Work out the finished part from the listing and answer in its coordinate system (mm). A direction names the side the tool comes from. Coordinates: 2 decimals unless noted, no trailing zeros. Loops run counter-clockwise (first coordinate to the right, second up) from the corner with the lowest first, then second, coordinate; pieces in that order, holes last. Notation, with made-up numbers: (-5.75, -33) - (43.25, -33) arc R14 ccw to (43.25, -6) - close; hole circle Ø2 at (42, -38). An arc over 180 degrees is marked (long way). Write each question's results on one line, items separated by ' | '. Start each with the question number.
Item 1: A tool of negligible diameter and unlimited length cuts with its end or side. For faces 1 (the face through (0, 1, -1)), 2 (the face through (0, 0, -3)), 3 (the face through (0, 1, 81)), from which of +Z, -Z, +X, -X, +Y, -Y can it reach the whole face along a straight path? Write none if from no direction.
Item 2: Each of these flat-tipped pins is pushed along its axis until it touches: pin 1 Ø1.5 at (x, z) = (-0.5, 46) entering from +Y; pin 2 Ø2 at (x, z) = (1.5, 39.5) entering from +Y. Where does it stop, or does it pass through?
Item 3: Section C-C, the plane z = 68.5 is taken. Write down the section's boundary in (x, y).
Item 4: Section A-A, the plane y = 0 is taken. Write down the section's boundary in (x, z), plus the area to 3 significant figures.
Item 5: Consider probe 1 along Z at (x, y) = (0.95, -1.05); probe 2 along X at (y, z) = (-0.15, 50). Determine where each line is inside the solid, lowest interval first. Write a range as [from, to].
Autodesk Inventor part; units mm, degrees
ref_plane "YZ Plane" through (0, 0, 0) normal (1, 0, 0) x (0, 1, 0)
ref_plane "XZ Plane" through (0, 0, 0) normal (0, 1, 0) x (-1, 0, 0)
ref_plane "XY Plane" through (0, 0, 0) normal (0, 0, 1) x (1, 0, 0)
sketch "Sketch1" plane through (0, 0, 0) normal (0, 0, 1) x (1, 0, 0)
  circle A0 centre (0, 0) radius 2.5
  dimension "d0" = 5
extrude "Extrusion1" add sketch "Sketch1" along normal blind 80
sketch "Sketch2" plane through (0, 0, 80) normal (0, 0, 1) x (1, 0, 0)
  circle A0 centre (0, 0) radius 2.5
  circle A1 centre (0, 0) radius 1
  dimension "d3" = 2
extrude "Extrusion2" add sketch "Sketch2" along normal blind 3 contours A1
sketch "Sketch3" plane through (0, 0, 0) normal (0, 0, -1) x (-1, 0, 0)
  circle A0 centre (0, 0) radius 1
  dimension "d6" = 2
extrude "Extrusion3" add sketch "Sketch3" along normal blind 3
properties part number "Bone-8cm"
Answer key:
1) face 1: -Z | face 2: -Z, +X, -X, +Y, -Y | face 3: +Z
2) pin 1: stops at y = 2.5 | pin 2: stops at y = 2.45
3) outline: circle Ø5 at (0, 0)
4) outline: (-2.5, 0) - (-1, 0) - (-1, -3) - (1, -3) - (1, 0) - (2.5, 0) - (2.5, 80) - (1, 80) - (1, 83) - (-1, 83) - (-1, 80) - (-2.5, 80) - close | area: 412 mm^2
5) probe 1: z = [0, 80] | probe 2: x = [-2.5, 2.5]
